Source: CAD feature listing. Evaluate the final solid. Frame: model axes, mm. A direction names the side the tool comes from. Give positions to 0.01 mm unless a question says otherwise; leave off trailing zeros. Write each loop counter-clockwise with the first axis right and the second up, starting at its lowest first coordinate (ties: lowest second). Pieces come first, ordered by that corner, then holes.
```python
from build123d import *

# Parameters (mm, degrees)
F1_DEPTH = 10
F2_R     = 1
F3_SIZE  = 0.5


with BuildPart() as f1:
    # F0 (on Front) → F1 (new body)
    with BuildSketch(Plane.XZ):
        Polygon((15, 0.4), (15, 2.5), (-14, 0.566667), (-14, 0), (-14, -0.566667), (15, -2.5), (15, -0.4), (7, -0.4), (7, 0.4), align=None)
    extrude(amount=F1_DEPTH)

    # F2
    f2_edges = [f1.edges().sort_by_distance(p)[0] for p in [
        (15, -5, -0.4),
        (15, -5, 0.4),
        (15, -5, -2.5),
        (15, -5, 2.5),
    ]]
    fillet(f2_edges, radius=F2_R)

    # F3
    f3_edges = [f1.edges().sort_by_distance(p)[0] for p in [
        (-14, -5, 0.566667),
        (-14, -5, -0.566667),
    ]]
    chamfer(f3_edges, length=F3_SIZE)


solid = f1.part
```
1. Section query A-A (x = 12.5). Return loops of the section in (y, z), plus the area to 3 significant figures.
2. Line query: probe 1 along Z at (x, y) = (9, -1); probe 2 along X at (y, z) = (-0.75, 0.3); probe 3 along Z at (x, y) = (-1.25, -0.75). Output: solid intervals per line, ascending.
3. Section query D-D (z = -1.15). Return loops of the section in (x, y), plus the area to 3 significant figures.
4. Pull-direction query (Z, two-part tool) for faces 3 (the flat face through (0.408, -4.93, 1.527)), 4 (the flat face through (0, -4.9, -1.5)), 5 (the flat face through (10, -5, 0.4)); classes: pulls with the +Z half, pulls with the -Z half, needs draft (parallel to the pull), parting line crosses it, or undercut.
5. Pin query (flat end, axial travel): P1, Ø5.5, axis at x = 9, y = -7.5, coming from the +Z side; P2, Ø4, axis at x = 9.5, y = -3.5, coming from the -Z side; P3, Ø6, axis at x = 4, y = -8.5, coming from the -Z side. Return the tip coordinate at first contact, or that it passes through.
6. Access query for faces 1 (the cylindrical face through (14.715, -5.07, -0.701)), 2 (the flat face through (4, 0, 0)). Directions: +Z, -Z, +X, -X, +Y, -Y. A direction counts if a zero-diameter tool reaches every point of the face in a straight line with its end or side. Return the directions, or none.
7. Section query C-C (x = 6.75). Return loops of the section in (y, z), plus the area to 3 significant figures.
The answers:
1. outline: (-10, -2.33) - (0, -2.33) - (0, -0.4) - (-10, -0.4) - close; (-10, 0.4) - (0, 0.4) - (0, 2.33) - (-10, 2.33) - close
1. area: 38.7 mm2
2. probe 1: z = -2.1 to -0.4, 0.4 to 2.1
2. probe 2: x = -13.78 to 7
2. probe 3: z = -1.42 to 1.42
3. outline: (-5.25, -10) - (14.97, -10) - (14.97, 0) - (-5.25, 0) - close
3. area: 202 mm2
4. face 3: pulls with the +Z half
4. face 4: pulls with the -Z half
4. face 5: undercut
5. P1: stops at z = 2.28
5. P2: stops at z = -2.27
5. P3: stops at z = -1.97
6. face 1: +X, +Y, -Y
6. face 2: +Z, -Z, +X, -X, +Y
7. outline: (-10, -1.95) - (0, -1.95) - (0, 1.95) - (-10, 1.95) - close
7. area: 39.0 mm2
